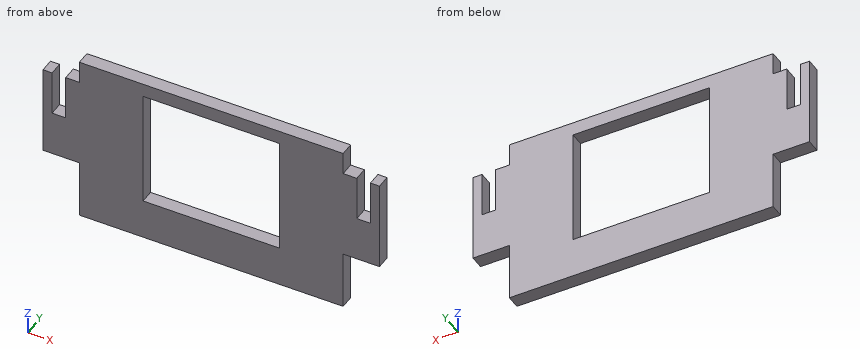
```python
from build123d import *

# Parameters (mm, degrees)
F0_W     = 30
F0_H     = 26
F1_DEPTH = 1.5


with BuildPart() as f1:
    # F0 (on Front) → F1 (new body, symmetric)
    with BuildSketch(Plane.XZ):
        Polygon((29, 28), (-29, 28), (-29, 23), (-32, 23), (-32, 13), (-35, 13), (-35, 23), (-37, 23), (-37, 3), (-29, 3), (-29, -10), (29, -10), (29, 3), (37, 3), (37, 23), (35, 23), (35, 13), (32, 13), (32, 23), (29, 23), align=None)
        with Locations((0, 12)):
            Rectangle(F0_W, F0_H, mode=Mode.SUBTRACT)
    extrude(amount=F1_DEPTH, both=True)


solid = f1.part
```
Build history of the part. All positions in model axes, mm. Give positions to 0.01 mm unless a question says otherwise; leave off trailing zeros. Loops run counter-clockwise (first coordinate to the right, second up) from the corner with the lowest first, then second, coordinate; pieces in that order, holes last. Notation, with made-up numbers: (-27, 44.25) -> (22, 44.25) arc R30 cw to (22, 73.25) -> close; hole circle Ø4 at (47.5, -39). An arc over 180 degrees is marked (long way). One line per question, with ' | ' between items.
Q1. Cut at B-B, the plane x = -6.5. Write the cut outline in (y, z).
Filled sheet:
outline: (-1.5, -10) -> (1.5, -10) -> (1.5, -1) -> (-1.5, -1) -> close; (-1.5, 25) -> (1.5, 25) -> (1.5, 28) -> (-1.5, 28) -> close
Q2. Cut at A-A, the plane z = 0. Write the cut outline in (x, y).
Filled sheet:
outline: (-29, -1.5) -> (-15, -1.5) -> (-15, 1.5) -> (-29, 1.5) -> close; (15, -1.5) -> (29, -1.5) -> (29, 1.5) -> (15, 1.5) -> close
Q3. Drop flat-ended pins along their axis: pin 1 (0.9 mm diameter, centred on y = -0.5, z = 25, fed in from +X); pin 2 (0.9 mm diameter, centred on x = -32.5, y = 0, fed in from -Z); pin 3 (1.5 mm diameter, centred on x = 33.5, y = -0.5, fed in from +Z). Give the stop position or say it passes through.
Filled sheet:
pin 1: stops at x = 29 | pin 2: stops at z = 3 | pin 3: stops at z = 13
Q4. Cut at D-D, the plane y = 0.2. Write the cut outline in (x, z), plus the area to 3 significant figures.
Filled sheet:
outline: (-37, 3) -> (-29, 3) -> (-29, -10) -> (29, -10) -> (29, 3) -> (37, 3) -> (37, 23) -> (35, 23) -> (35, 13) -> (32, 13) -> (32, 23) -> (29, 23) -> (29, 28) -> (-29, 28) -> (-29, 23) -> (-32, 23) -> (-32, 13) -> (-35, 13) -> (-35, 23) -> (-37, 23) -> close; hole (-15, -1) -> (15, -1) -> (15, 25) -> (-15, 25) -> close | area: 1,680 mm²
Q5. Drill centre lines: line 1 along X through (y, z) = (1.4, 17.5); line 2 along X through (y, z) = (-0.7, 0); line 3 along Z through (x, y) = (10.5, -0.1). Where is each one in solid material? Low to high. Write a range as [from, to].
Filled sheet:
line 1: x = [-37, -35], [-32, -15], [15, 32], [35, 37] | line 2: x = [-29, -15], [15, 29] | line 3: z = [-10, -1], [25, 28]
Q6. Cut at C-C, the plane z = 16.5. Write the cut outline in (x, y).
Filled sheet:
outline: (-37, -1.5) -> (-35, -1.5) -> (-35, 1.5) -> (-37, 1.5) -> close; (-32, -1.5) -> (-15, -1.5) -> (-15, 1.5) -> (-32, 1.5) -> close; (15, -1.5) -> (32, -1.5) -> (32, 1.5) -> (15, 1.5) -> close; (35, -1.5) -> (37, -1.5) -> (37, 1.5) -> (35, 1.5) -> close
